from build123d import *

# Parameters (mm, degrees)
O_L_DEPTH             = 17.85
CUT_EXTRUDE4_REACH    = 17
CUT_EXTRUDE2_REACH    = 13.95
SKETCH4_R             = 3
CHAMFER4_SIZE         = 0.5
M5_TAPPED_HOLE1_D     = 4.2
M5_TAPPED_HOLE1_DEPTH = 6
M5_TAPPED_HOLE1_TIP   = 1.212435565


with BuildPart() as part:
    # Sketch1 → Revolve1 (revolve)
    with BuildSketch(Plane.XY):
        with BuildLine():
            Line((-22, 0), (-22, 5))
            Line((-22, 5), (-21, 6))
            Line((-21, 6), (-11.125, 6))
            Line((-11.125, 6), (-11.058578644, 5.933578644))
            ThreePointArc((-11.058578644, 5.933578644), (-10.993693974, 5.890224093), (-10.917157288, 5.875))
            Line((-10.917157288, 5.875), (-10.2, 5.875))
            ThreePointArc((-10.2, 5.875), (-10.058578644, 5.933578644), (-10, 6.075))
            Line((-10, 6.075), (-10, 9))
            Line((-10, 9), (0, 9))
            Line((0, 9), (0, 5.75))
            Line((0, 5.75), (1.35, 5.75))
            Line((1.35, 5.75), (1.35, 4.25))
            Line((1.35, 4.25), (1.75, 4.25))
            Line((1.75, 4.25), (2.55, 5.05))
            Line((2.55, 5.05), (4.238756443, 5.05))
            Line((4.238756443, 5.05), (4.5, 4.98))
            Line((4.5, 4.98), (4.8, 4.98))
            Line((4.8, 4.98), (5, 4.78))
            Line((5, 4.78), (5, 0))
            Line((5, 0), (-22, 0))
        make_face()
    revolve(axis=Axis((0, 0, 0), (1, 0, 0)))

    # Sketch3 → O-L (cut)
    with BuildSketch(Plane.ZY.offset(22)):
        with BuildLine():
            Line((-4, 8.062257748), (-4, -8.062257748))
            ThreePointArc((-4, -8.062257748), (-9, 0), (-4, 8.062257748))
        make_face()
        with BuildLine():
            Line((4, 8.062257748), (4, -8.062257748))
            ThreePointArc((4, -8.062257748), (9, 0), (4, 8.062257748))
        make_face()
    extrude(amount=-O_L_DEPTH, mode=Mode.SUBTRACT)

    # Sketch6 → Cut-Extrude4 (cut, up to next)
    with BuildSketch(Plane.ZY.offset(10), mode=Mode.PRIVATE) as cut_extrude4_sk1:
        with BuildLine():
            Line((-4.218708333, 7.95), (4.218708333, 7.95))
            ThreePointArc((4.218708333, 7.95), (0, 9), (-4.218708333, 7.95))
        make_face()
    cut_extrude4_tool1 = extrude(cut_extrude4_sk1.sketch, amount=-CUT_EXTRUDE4_REACH, mode=Mode.PRIVATE) & part.part
    add(cut_extrude4_tool1.solids().sort_by_distance((-10, 8.372173, 0))[0], mode=Mode.SUBTRACT)
    # Sketch6 → Cut-Extrude4 (cut, up to next)
    with BuildSketch(Plane.ZY.offset(10), mode=Mode.PRIVATE) as cut_extrude4_sk2:
        with BuildLine():
            Line((7.95, 4.218708333), (7.95, -4.218708333))
            ThreePointArc((7.95, -4.218708333), (9, 0), (7.95, 4.218708333))
        make_face()
    cut_extrude4_tool2 = extrude(cut_extrude4_sk2.sketch, amount=-CUT_EXTRUDE4_REACH, mode=Mode.PRIVATE) & part.part
    add(cut_extrude4_tool2.solids().sort_by_distance((-10, 0, 8.372173))[0], mode=Mode.SUBTRACT)
    # Sketch6 → Cut-Extrude4 (cut, up to next)
    with BuildSketch(Plane.ZY.offset(10), mode=Mode.PRIVATE) as cut_extrude4_sk3:
        with BuildLine():
            Line((4.218708333, -7.95), (-4.218708333, -7.95))
            ThreePointArc((-4.218708333, -7.95), (0, -9), (4.218708333, -7.95))
        make_face()
    cut_extrude4_tool3 = extrude(cut_extrude4_sk3.sketch, amount=-CUT_EXTRUDE4_REACH, mode=Mode.PRIVATE) & part.part
    add(cut_extrude4_tool3.solids().sort_by_distance((-10, -8.372173, 0))[0], mode=Mode.SUBTRACT)
    # Sketch6 → Cut-Extrude4 (cut, up to next)
    with BuildSketch(Plane.ZY.offset(10), mode=Mode.PRIVATE) as cut_extrude4_sk4:
        with BuildLine():
            Line((-7.95, -4.218708333), (-7.95, 4.218708333))
            ThreePointArc((-7.95, 4.218708333), (-9, 0), (-7.95, -4.218708333))
        make_face()
    cut_extrude4_tool4 = extrude(cut_extrude4_sk4.sketch, amount=-CUT_EXTRUDE4_REACH, mode=Mode.PRIVATE) & part.part
    add(cut_extrude4_tool4.solids().sort_by_distance((-10, 0, -8.372173))[0], mode=Mode.SUBTRACT)

    # Sketch4 → Cut-Extrude2 (cut, up to next)
    with BuildSketch(Plane.XY.offset(4), mode=Mode.PRIVATE) as cut_extrude2_sk1:
        with Locations((-12, 0)):
            Circle(SKETCH4_R)
    cut_extrude2_tool1 = extrude(cut_extrude2_sk1.sketch, amount=-CUT_EXTRUDE2_REACH, mode=Mode.PRIVATE) & part.part
    add(cut_extrude2_tool1.solids().sort_by_distance((-12, 0, 4))[0], mode=Mode.SUBTRACT)

    # Chamfer4
    chamfer4_edges = [part.edges().sort_by_distance(p)[0] for p in [
        (-15, 0, 4),
        (-15, 0, -4),
    ]]
    chamfer(chamfer4_edges, length=CHAMFER4_SIZE)

    # M5 Tapped Hole1
    with Locations(Plane(origin=(0, 7.95, 0), x_dir=(1, 0, 0), z_dir=(0, 1, 0))):
        with Locations((-4, 0)):
            Hole(M5_TAPPED_HOLE1_D / 2, depth=M5_TAPPED_HOLE1_DEPTH)
            with Locations((0, 0, -(M5_TAPPED_HOLE1_DEPTH + M5_TAPPED_HOLE1_TIP / 2))):  # 120° drill point
                Cone(0, M5_TAPPED_HOLE1_D / 2, M5_TAPPED_HOLE1_TIP, mode=Mode.SUBTRACT)


solid = part.part
The listing builds one solid part. Answer for the finished solid, in the listing's coordinates (mm). A direction names the side the tool comes from. Give positions to 0.01 mm unless a question says otherwise; leave off trailing zeros. Write each loop counter-clockwise with the first axis right and the second up, starting at its lowest first coordinate (ties: lowest second). Pieces come first, ordered by that corner, then holes.
Item 1: Section A-A, the plane x = -12 is taken. Write down the section's boundary in (y, z), plus the area to 3 significant figures.
Item 2: Section C-C, the plane x = 0.75 is taken. Write down the section's boundary in (y, z), plus the area to 3 significant figures.
Item 3: Flat-ended cylindrical pins translate along their axes: P1, Ø3, axis at x = -8, z = 5, coming from the +Y side; P2, Ø5, axis at x = -13, y = 2.5, coming from the -Z side; P3, Ø3, axis at y = -3.5, z = 6, coming from the -X side; P4, Ø8, axis at x = -12, y = 0, coming from the +Z side. Find the tip coordinate at first contact, or state that the pin passes through.
Item 4: Determine the mould class of faces 1 (the flat face through (-2, 0, 7.95)), 2 (the flat face through (-22, 0, 0)), 3 (the flat face through (0, -4, 5)), 4 (the cylindrical face through (-10.554, 5.875, -0.062)) for opening direction X: released by +X, released by -X, zero draft, split by the parting line, or undercut.
Item 5: Which of the six approach directions +Z, -Z, +X, -X, +Y, -Y give full straight-line access (tool end or side, diameter ignored) to faces 5 (the cylindrical face through (-16, -6, 0)), 6 (the flat face through (-11, 4, -4)), 7 (the cylindrical face through (1.553, 2.285, 3.584)), 8 (the flat face through (-11, 4, 4)), 9 (the conical face through (-21.8, 5.2, -0.1))?
Item 6: Find the intervals of material crossed by line 1 along X through (y, z) = (1.5, 0.5); line 2 along X through (y, z) = (5.5, -5.5); line 3 along Z through (x, y) = (-4, 4.5), in increasing order.
Completed:
1. outline: (-4.47, -4) - (-3.5, -4) - (-3, -3.5) - (-3, 3.5) - (-3.5, 4) - (-4.47, 4) arc R6 ccw to start; (3, -3.5) - (3.5, -4) - (4.47, -4) arc R6 ccw to (4.47, 4) - (3.5, 4) - (3, 3.5) - close
1. area: 39.8 mm2
2. outline: circle Ø11.5 at (0, 0)
2. area: 104 mm2
3. P1: stops at y = 7.95
3. P2: stops at z = -4
3. P3: stops at x = -4.15
3. P4: stops at z = 4
4. face 1: zero draft
4. face 2: released by -X
4. face 3: released by +X
4. face 4: undercut
5. face 5: -X, -Y
5. face 6: -Z, -X, +Y, -Y
5. face 7: none
5. face 8: +Z, -X, +Y, -Y
5. face 9: -X, +Y
6. line 1: x = -22 to -14.6, -9.4 to -5.22, -2.78 to 5
6. line 2: x = -4.15 to 0
6. line 3: z = -7.79 to -2.1, 2.1 to 7.79
